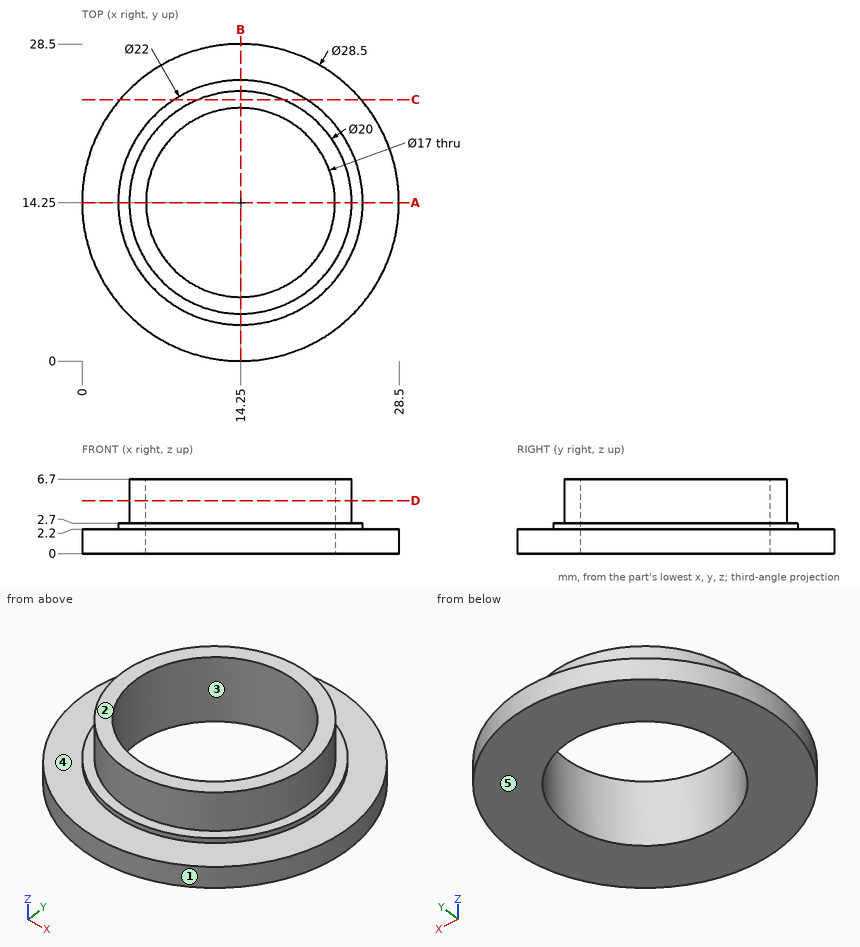
Could you check a few things on this drawing? It's one solid part, dimensions in mm from its lowest x, y, z. A direction names the side the tool comes from. Give positions to 0.01 mm unless a question says otherwise; leave off trailing zeros. Loops run counter-clockwise (first coordinate to the right, second up) from the corner with the lowest first, then second, coordinate; pieces in that order, holes last. Notation, with made-up numbers: (72, 68) -> (103, 68) arc R37 ccw to (103, 105) -> close; hole circle Ø6 at (87, 17). An arc over 180 degrees is marked (long way). Answer as CSV lines item,"result". Start each with the question number.
(1) If we section it at C-C on y = 23.5: Write out the boundary of the cut face in (x, z).
(2) We'd pull the mould along X, two halves only. Please class the marked faces 1, 2 and 3: released by +X, released by -X, zero draft, split by the parting line, or undercut.
(3) If we section it at D-D on z = 4.75: Write out the boundary of the cut face in (x, y).
(4) Which directions (+Z, -Z, +X, -X, +Y, -Y) give clear straight access to the entire face, cutting with the end or side of a thin tool? Please do the marked faces 4 and 5.
(5) I need wall thicknesses on probe 1 along Y at (x, z) = (14.25, 1.5); probe 2 along Y at (x, z) = (14.25, 4.75). Which ranges of each line are inside material? Lowest first, please.
(6) If we section it at A-A on y = 14.25: Write out the boundary of the cut face in (x, z), then the cut area to 3 significant figures.
(7) I'm going to push a flat-ended pin straight in: pin 1 Ø1.5 at (x, z) = (17, 5.5) entering from -Y. Where does the tip first touch, or does it pass through?
Computed:
1,outline,"(3.41, 0) -> (25.09, 0) -> (25.09, 2.2) -> (20.2, 2.2) -> (20.2, 2.7) -> (18.05, 2.7) -> (18.05, 6.7) -> (10.45, 6.7) -> (10.45, 2.7) -> (8.3, 2.7) -> (8.3, 2.2) -> (3.41, 2.2) -> close"
2,face 1,"split by the parting line"
2,face 2,"zero draft"
2,face 3,"undercut"
3,outline,"circle Ø20 at (14.25, 14.25); hole circle Ø17 at (14.25, 14.25)"
4,face 4,"+Z"
4,face 5,"-Z, +X, -X, +Y, -Y"
5,probe 1,"y = 0 to 5.75, 22.75 to 28.5"
5,probe 2,"y = 4.25 to 5.75, 22.75 to 24.25"
6,outline,"(0, 0) -> (5.75, 0) -> (5.75, 6.7) -> (4.25, 6.7) -> (4.25, 2.7) -> (3.25, 2.7) -> (3.25, 2.2) -> (0, 2.2) -> close; (22.75, 0) -> (28.5, 0) -> (28.5, 2.2) -> (25.25, 2.2) -> (25.25, 2.7) -> (24.25, 2.7) -> (24.25, 6.7) -> (22.75, 6.7) -> close"
6,area,"39.8 mm2"
7,pin 1,"stops at y = 4.45"
